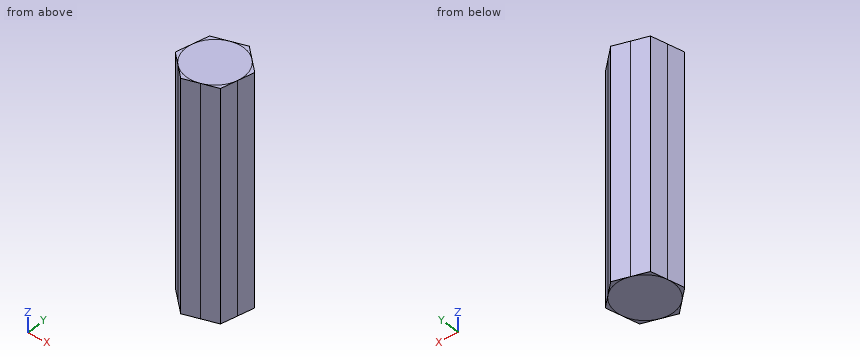
Autodesk Inventor part; units mm, degrees
ref_plane "YZ Plane" through (0, 0, 0) normal (1, 0, 0) x (0, 1, 0)
ref_plane "XZ Plane" through (0, 0, 0) normal (0, 1, 0) x (-1, 0, 0)
ref_plane "XY Plane" through (0, 0, 0) normal (0, 0, 1) x (1, 0, 0)
sketch "Sketch1" plane through (0, 0, 0) normal (0, 0, 1) x (1, 0, 0)
  circle A0 centre (0, 0) radius 6.35
  line L0 (6.9674, 2.2843) -> (5.462, -4.8918)
  line L1 (5.462, -4.8918) -> (-1.5054, -7.1761)
  line L2 (-1.5054, -7.1761) -> (-6.9674, -2.2843)
  line L3 (-6.9674, -2.2843) -> (-5.462, 4.8918)
  line L4 (-5.462, 4.8918) -> (1.5054, 7.1761)
  line L5 (1.5054, 7.1761) -> (6.9674, 2.2843)
  point P0 (4.2364, 4.7302)
  dimension "d0" = 12.7
extrude "Extrusion1" add sketch "Sketch1" along normal blind 50.8
properties part number "4-bar intake (2) shaft"
Design review of the part built by this model. Coordinates are the model's own, in mm. Coordinates: 2 decimals unless noted, no trailing zeros. Loops run counter-clockwise (first coordinate to the right, second up) from the corner with the lowest first, then second, coordinate; pieces in that order, holes last. Notation, with made-up numbers: (22.25, 11.25) - (44.25, 11.25) arc R21 cw to (44.25, 40.25) - close; hole circle Ø4 at (76.25, 18). An arc over 180 degrees is marked (long way). Use CSV: the item, a comma, the result in double quotes. Start each with the question number.
1. To check wall thickness, follow probe 1 along Y at (x, z) = (1.5, 41); probe 2 along X at (y, z) = (-4.25, 26); probe 3 along X at (y, z) = (-2, 35.5). State the ranges of each line that lie inside material, in increasing order.
2. Add section C-C on x = 3.25. Give the boundary of the cut face in (y, z), plus the area to 3 significant figures.
3. Add section A-A on z = 17.5. Give the boundary of the cut face in (x, y), plus the area to 3 significant figures.
4. Clearance check with flat-ended pins moving along their axes: pin 1 (5 mm diameter, centred on x = 4, z = 19, fed in from -Y); pin 2 (3 mm diameter, centred on x = 3.5, z = 9.5, fed in from -Y); pin 3 (2 mm diameter, centred on x = -1.5, z = 34.5, fed in from +Y). State where each tip first meets the part, or that it passes through.
5. Add section B-B on y = 3. Give the boundary of the cut face in (x, z).
Resolved:
1,probe 1,"-6.19 to 7.17"
1,probe 2,"-4.77 to 5.6"
1,probe 3,"-6.91 to 6.07"
2,outline,"(-5.62, 0) - (5.61, 0) - (5.61, 50.8) - (-5.62, 50.8) - close"
2,area,"571 mm2"
3,outline,"(-6.97, -2.28) - (-1.51, -7.18) - (5.46, -4.89) - (6.97, 2.28) - (1.51, 7.18) - (-5.46, 4.89) - close"
3,area,"140 mm2"
4,pin 1,"y = -6.19"
4,pin 2,"y = -6.03"
4,pin 3,"y = 6.52"
5,outline,"(-5.86, 0) - (6.17, 0) - (6.17, 50.8) - (-5.86, 50.8) - close"
